Part model, mm, in its own coordinate system. Face numbers are marked on the shaded views. Coordinates: 2 decimals unless noted, no trailing zeros. Order: outer loops, then holes, each group sorted by start corner. A loop starts at its lowest first (then second) coordinate and runs counter-clockwise, first axis right, second up. Notation, with made-up numbers: (-19, 58.25) - (40, 58.25) arc R16 ccw to (40, 78.25) - close; hole circle Ø3 at (49.25, 77.25). An arc over 180 degrees is marked (long way). Use a Markdown table: item, result. Add a question column.
1) Drop flat-ended pins along their axis: P1, Ø1.1, axis at x = 3.5, y = 79.5, coming from the +Z side; P2, Ø12, axis at x = -42, y = 69, coming from the +Z side; P3, Ø1.8, axis at x = 3, y = 80.5, coming from the -Z side. Give the stop position or say it passes through.
2) Wall check: L1, parallel to X at y = 79, z = 0; L2, parallel to X at y = 44.5, z = 0. Give the ranges that are in metal, low to high. Write a range as [from, to].
3) Saw through at B-B on y = 27.5. List the corners of the cut face in (x, z).
4) Two-plate mould, pull along Z, no slides. Class the marked faces 1, 2 and 3: +Z half, -Z half, draft (parallel to the pull), parting line (faces both ways), or undercut.
5) Saw through at A-A on y = 86.5. List the corners of the cut face in (x, z), then the cut area to 3 significant figures.
```python
from build123d import *

# Parameters (mm, degrees)
SKETCH1_R           = 83.82
BOSS_EXTRUDE1_DEPTH = 127
SHELL1_T            = -6.35
CUT_EXTRUDE2_REACH  = 146.451
FILLET2_R           = 2.54


with BuildPart() as part:
    # Sketch1 → Boss-Extrude1 (new body)
    with BuildSketch(Plane(origin=(0, 0, 0), x_dir=(1, 0, 0), z_dir=(0, 1, 0))):
        with Locations(Location((0, 0, 0), (0, 0, 270))):
            Circle(SKETCH1_R)
    extrude(amount=BOSS_EXTRUDE1_DEPTH)

    # Sketch2 → Cut-Revolve1 (revolve, cut)
    with BuildSketch(Plane.XY, mode=Mode.PRIVATE) as cut_revolve1_sk:
        Polygon((-5.08, 82.55), (0, 82.55), (0, 127), (-71.12, 127), align=None)
    revolve(cut_revolve1_sk.sketch.rotate(Axis((0, 0, 0), (0, 1, 0)), 90), axis=Axis((0, 0, 0), (0, 1, 0)), mode=Mode.SUBTRACT)

    # Shell1
    shell1_openings = [part.faces().sort_by_distance(p)[0] for p in [
        (0, 0, 0),
    ]]
    offset(amount=SHELL1_T, openings=shell1_openings, kind=Kind.INTERSECTION)

    # Sketch4 → Cut-Extrude2 (cut, up to next)
    with BuildSketch(Plane(origin=(0, 82.55, 0), x_dir=(1, 0, 0), z_dir=(0, 1, 0)), mode=Mode.PRIVATE) as cut_extrude2_sk1:
        with BuildLine():
            Line((-1.27, 1.27), (-1.27, 4.91868885))
            ThreePointArc((-1.27, 4.91868885), (-3.592102448, 3.592102448), (-4.91868885, 1.27))
            Line((-4.91868885, 1.27), (-1.27, 1.27))
        make_face()
    cut_extrude2_tool1 = extrude(cut_extrude2_sk1.sketch, amount=-CUT_EXTRUDE2_REACH, mode=Mode.PRIVATE) & part.part
    # Sketch4 → Cut-Extrude2 (cut, up to next)
    with BuildSketch(Plane(origin=(0, 82.55, 0), x_dir=(1, 0, 0), z_dir=(0, 1, 0)), mode=Mode.PRIVATE) as cut_extrude2_sk2:
        with BuildLine():
            ThreePointArc((4.91868885, 1.27), (3.592102448, 3.592102448), (1.27, 4.91868885))
            Line((1.27, 4.91868885), (1.27, 1.27))
            Line((1.27, 1.27), (4.91868885, 1.27))
        make_face()
    cut_extrude2_tool2 = extrude(cut_extrude2_sk2.sketch, amount=-CUT_EXTRUDE2_REACH, mode=Mode.PRIVATE) & part.part
    # Sketch4 → Cut-Extrude2 (cut, up to next)
    with BuildSketch(Plane(origin=(0, 82.55, 0), x_dir=(1, 0, 0), z_dir=(0, 1, 0)), mode=Mode.PRIVATE) as cut_extrude2_sk3:
        with BuildLine():
            Line((-1.27, -4.91868885), (-1.27, -1.27))
            Line((-1.27, -1.27), (-4.91868885, -1.27))
            ThreePointArc((-4.91868885, -1.27), (-3.592102448, -3.592102448), (-1.27, -4.91868885))
        make_face()
    cut_extrude2_tool3 = extrude(cut_extrude2_sk3.sketch, amount=-CUT_EXTRUDE2_REACH, mode=Mode.PRIVATE) & part.part
    # Sketch4 → Cut-Extrude2 (cut, up to next)
    with BuildSketch(Plane(origin=(0, 82.55, 0), x_dir=(1, 0, 0), z_dir=(0, 1, 0)), mode=Mode.PRIVATE) as cut_extrude2_sk4:
        with BuildLine():
            Line((4.91868885, -1.27), (1.27, -1.27))
            Line((1.27, -1.27), (1.27, -4.91868885))
            ThreePointArc((1.27, -4.91868885), (3.592102448, -3.592102448), (4.91868885, -1.27))
        make_face()
    cut_extrude2_tool4 = extrude(cut_extrude2_sk4.sketch, amount=-CUT_EXTRUDE2_REACH, mode=Mode.PRIVATE) & part.part
    add(cut_extrude2_tool1.solids().sort_by_distance((-2.704204, 82.55, -2.704204))[0], mode=Mode.SUBTRACT)
    add(cut_extrude2_tool2.solids().sort_by_distance((2.704204, 82.55, -2.704204))[0], mode=Mode.SUBTRACT)
    add(cut_extrude2_tool3.solids().sort_by_distance((-2.704204, 82.55, 2.704204))[0], mode=Mode.SUBTRACT)
    add(cut_extrude2_tool4.solids().sort_by_distance((2.704204, 82.55, 2.704204))[0], mode=Mode.SUBTRACT)

    # Fillet2
    fillet2_edges = [part.edges().sort_by_distance(p)[0] for p in [
        (0, 127, -83.82),
    ]]
    fillet(fillet2_edges, radius=FILLET2_R)


solid = part.part
```
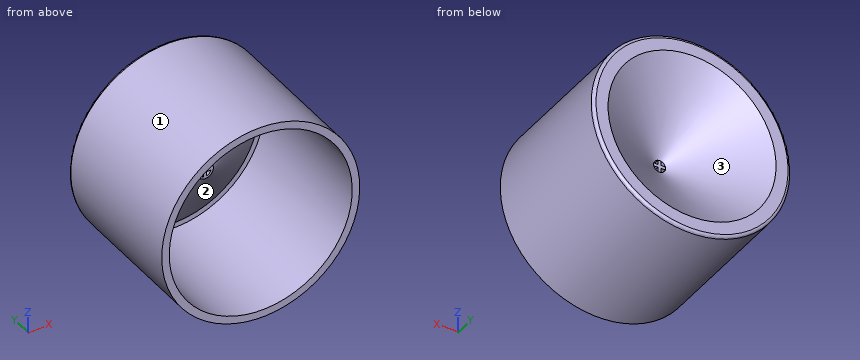
Results are:
| question | item | result |
|---|---|---|
| 1 | P1 | z = 83.77 |
| 1 | P2 | z = 75.7 |
| 1 | P3 | z = -83.79 |
| 2 | L1 | [-83.82, -77.47], [-11.18, 11.18], [77.47, 83.82] |
| 2 | L2 | [-83.82, -77.47], [77.47, 83.82] |
| 3 | outline | circle Ø167.64 at (0, 0); hole circle Ø154.94 at (0, 0) |
| 4 | face 1 | parting line |
| 4 | face 2 | undercut |
| 4 | face 3 | undercut |
| 5 | outline | circle Ø167.64 at (0, 0); circle Ø44.64 at (0, 0); hole circle Ø154.94 at (0, 0); hole circle Ø21.9 at (0, 0) |
| 5 | area | 4,410 mm2 |
